Input: part model. Units: mm. Frame: model coordinates. A direction names the side the tool comes from. Coordinates: 2 decimals unless noted, no trailing zeros. Loops run counter-clockwise (first coordinate to the right, second up) from the corner with the lowest first, then second, coordinate; pieces in that order, holes last. Notation, with made-up numbers: (-20, 64.25) - (33, 64.25) arc R18 cw to (33, 95.25) - close; hole circle Ø1 at (64.25, 30.5). An arc over 180 degrees is marked (long way). Use one line per item in the form item = value.
from build123d import *

# Parameters (mm, degrees)
SKETCH1_W                           = 32
SKETCH1_H                           = 30
BOSS_EXTRUDE1_DEPTH                 = 3
BOSS_EXTRUDE2_DEPTH                 = 3
F_1_5MM_CLEARANCE_DOWEL_HOLE1_D     = 1.5
F_1_5MM_CLEARANCE_DOWEL_HOLE1_DEPTH = 5
F_1_5MM_CLEARANCE_DOWEL_HOLE1_TIP   = 0.450645464
FILLET1_R                           = 5
FILLET2_R                           = 3.5
BOSS_EXTRUDE4_DEPTH                 = 32
BOSS_EXTRUDE5_DEPTH                 = 32
SKETCH8_R                           = 1.25
CUT_EXTRUDE1_DEPTH                  = 7.503603871
FILLET3_R                           = 1
FILLET4_R                           = 2
FILLET5_R                           = 1


with BuildPart() as part:
    # Sketch1 → Boss-Extrude1 (new body)
    with BuildSketch(Plane.XY):
        with Locations((16, 15)):
            Rectangle(SKETCH1_W, SKETCH1_H)
    extrude(amount=BOSS_EXTRUDE1_DEPTH)

    # Sketch2 → Boss-Extrude2 (add)
    with BuildSketch(Plane.XY.offset(3)):
        with BuildLine():
            Line((1.5, 0), (3.3, 0))
            Line((3.3, 0), (3.3, 10))
            Line((3.3, 10), (5.5, 10))
            ThreePointArc((5.5, 10), (8, 12.5), (5.5, 15))
            Line((5.5, 15), (3.3, 15))
            Line((3.3, 15), (3.3, 22.5))
            Line((3.3, 22.5), (5.5, 22.5))
            ThreePointArc((5.5, 22.5), (7.267766953, 23.232233047), (8, 25))
            Line((8, 25), (8, 26.7))
            Line((8, 26.7), (24, 26.7))
            Line((24, 26.7), (24, 25))
            ThreePointArc((24, 25), (24.732233047, 23.232233047), (26.5, 22.5))
            Line((26.5, 22.5), (28.7, 22.5))
            Line((28.7, 22.5), (28.7, 15))
            Line((28.7, 15), (26.5, 15))
            ThreePointArc((26.5, 15), (24, 12.5), (26.5, 10))
            Line((26.5, 10), (28.7, 10))
            Line((28.7, 10), (28.7, 0))
            Line((28.7, 0), (30.5, 0))
            Line((30.5, 0), (30.5, 28.5))
            Line((30.5, 28.5), (1.5, 28.5))
            Line((1.5, 28.5), (1.5, 0))
        make_face()
    extrude(amount=BOSS_EXTRUDE2_DEPTH)

    # Ø1.5mm Clearance Dowel Hole1
    with Locations(Plane(origin=(5.5, 25, 6), x_dir=(1, 0, 0), z_dir=(0, 0, 1))):
        with Locations((0, 0), (21, 0), (21, -12.5), (0, -12.5)):
            Hole(F_1_5MM_CLEARANCE_DOWEL_HOLE1_D / 2, depth=F_1_5MM_CLEARANCE_DOWEL_HOLE1_DEPTH)
            with Locations((0, 0, -(F_1_5MM_CLEARANCE_DOWEL_HOLE1_DEPTH + F_1_5MM_CLEARANCE_DOWEL_HOLE1_TIP / 2))):  # 118° drill point
                Cone(0, F_1_5MM_CLEARANCE_DOWEL_HOLE1_D / 2, F_1_5MM_CLEARANCE_DOWEL_HOLE1_TIP, mode=Mode.SUBTRACT)

    # Fillet1
    fillet1_edges = [part.edges().sort_by_distance(p)[0] for p in [
        (0, 30, 1.5),
        (32, 30, 1.5),
    ]]
    fillet(fillet1_edges, radius=FILLET1_R)

    # Fillet2
    fillet2_edges = [part.edges().sort_by_distance(p)[0] for p in [
        (1.5, 28.5, 4.5),
        (30.5, 28.5, 4.5),
    ]]
    fillet(fillet2_edges, radius=FILLET2_R)

    # Sketch5 → Boss-Extrude4 (add)
    with BuildSketch(Plane.ZY):
        Polygon((0, 0), (-7.243852416, 2.636546661), (-6.217791986, 5.455624523), (0, 3.192533317), align=None)
    extrude(amount=-BOSS_EXTRUDE4_DEPTH)

    # Sketch7 → Boss-Extrude5 (add)
    with BuildSketch(Plane.ZY):
        Polygon((0, 0), (3, -1.091910703), (3, 0), align=None)
    extrude(amount=-BOSS_EXTRUDE5_DEPTH)

    # Sketch8 → Cut-Extrude1 (cut, through all)
    with BuildSketch(Plane(origin=(0, 2.819077862, 1.02606043), x_dir=(1, 0, 0), z_dir=(0, 0.939692621, 0.342020143))):
        with Locations((4.810584477, 5.708746728)):
            Circle(SKETCH8_R)
        with Locations((27.189415523, 5.708746728)):
            Circle(SKETCH8_R)
    extrude(amount=-CUT_EXTRUDE1_DEPTH, mode=Mode.SUBTRACT)

    # Fillet3
    fillet3_edges = [part.edges().sort_by_distance(p)[0] for p in [
        (3.3, 10, 4.5),
        (3.3, 15, 4.5),
        (3.3, 22.5, 4.5),
        (8, 26.7, 4.5),
        (24, 26.7, 4.5),
        (28.7, 22.5, 4.5),
        (28.7, 15, 4.5),
        (28.7, 10, 4.5),
    ]]
    fillet(fillet3_edges, radius=FILLET3_R)

    # Fillet4
    fillet4_edges = [part.edges().sort_by_distance(p)[0] for p in [
        (16, 3.192533317, 0),
    ]]
    fillet(fillet4_edges, radius=FILLET4_R)

    # Fillet5
    fillet5_edges = [part.edges().sort_by_distance(p)[0] for p in [
        (0, 4.046085592, -6.730822201),
        (32, 4.046085592, -6.730822201),
    ]]
    fillet(fillet5_edges, radius=FILLET5_R)


solid = part.part
Q1. Pull-direction query (X, two-part tool) for faces 4 (the cylindrical face through (29.5, 27.45, 4.52)), 5 (the cylindrical face through (7, 23, 4)), 6 (the conical face through (26.624, 12.539, 0.628)), 7 (the flat face through (30, 0, 4)); classes: pulls with the +X half, pulls with the -X half, needs draft (parallel to the pull), parting line crosses it, or undercut.
Check values:
face_4 = pulls with the +X half
face_5 = undercut
face_6 = undercut
face_7 = needs draft
Q2. Set-up query: faces 1 (the flat face through (15.776, 4.822, -4.476)), 2 (the flat face through (3.3, 19, 4)), 3 (the flat face through (1.5, 13, 4)). Return all of +Z, -Z, +X, -X, +Y, -Y with unobstructed straight access to the full face (end or side cutting, diameter ignored); none if empty.
Check values:
face_1 = +X, -X, +Y
face_2 = +Z
face_3 = +Z, -X, +Y, -Y
Q3. Ray query, line 1 along X through (y, z) = (25, 3.3); line 2 along Y through (x, z) = (5.5, 4.45); line 3 along X through (y, z) = (12.5, 2.35). Return the intervals inside material, ascending. Write a range as [from, to].
Check values:
line_1 = [1.5, 4.75], [6.25, 8], [24, 25.75], [27.25, 30.5]
line_2 = [10, 11.75], [13.25, 15], [22.5, 24.25], [25.75, 28.5]
line_3 = [0, 4.75], [6.25, 25.75], [27.25, 32]
Q4. Cut plane D-D, the plane z = -1.75. Return loops of the section in (x, y).
Check values:
outline = (0, 0.64) - (32, 0.64) - (32, 4.06) - (0, 4.06) - close
Q5. Cut plane B-B, the plane y = 11. Return loops of the section in (x, z).
Check values:
outline = (0, 0) - (32, 0) - (32, 3) - (30.5, 3) - (30.5, 6) - (24.5, 6) - (24.5, 3) - (7.5, 3) - (7.5, 6) - (1.5, 6) - (1.5, 3) - (0, 3) - close
Q6. Cut plane A-A, the plane x = 18. Return loops of the section in (y, z), then the cut area to 3 significant figures.
Check values:
outline = (-1.09, 3) - (2.64, -7.24) - (5.46, -6.22) - (4.17, -2.68) arc R2 cw to (6.05, 0) - (30, 0) - (30, 3) - (28.5, 3) - (28.5, 6) - (26.7, 6) - (26.7, 3) - close
area = 120 mm²
Q7. Cut plane C-C, the plane z = 5.25. Give the number of separate pieces and of enclosed holes in the cut face, then the cut area to 3 significant figures.
Check values:
separate_pieces = 1
enclosed_holes = 4
area = 216 mm²
Q8. First-contact query: P1, Ø4, axis at x = 11.5, z = -3.5, coming from the -Y side; P2, Ø1.5, axis at x = 19, z = 4.5, coming from the +Y side; P3, Ø1.5, axis at y = 4, z = 4.5, coming from the +X side. Flat tips, straight axial feed; report the tip coordinate or a pass-through.
Check values:
P1 = 0.55
P2 = 28.5
P3 = 30.5
